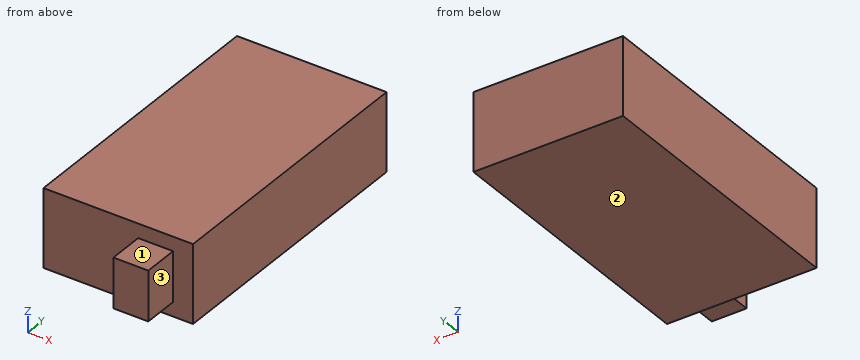
Autodesk Inventor part; units mm, degrees
ref_plane "Work Plane1" through (15.0814, 10.922, 0) normal (0, -1, 0) x (0, 0, -1)
ref_plane "XZ Plane" through (0, 0, 0) normal (0, 1, 0) x (-1, 0, 0)
sketch "Sketch1" plane through (0, 0, 0) normal (0, 0, 1) x (1, 0, 0)
  circle A0 centre (0, 0) radius 3.175
  line L0 (5.0349, -7.366) -> (-5.0349, -7.366)
  line L1 (-8.89, 10.922) -> (-8.89, -7.366)
  line L2 (8.89, -7.366) -> (8.89, 10.922)
  line L3 (-37.211, 10.922) -> (12.7, 10.922) construction
  line L4 (-8.89, 10.922) -> (8.89, 10.922)
  line L5 (8.89, 10.922) -> (8.89, -7.366)
  line L6 (8.89, -7.366) -> (-8.89, -7.366)
  line L7 (-8.89, -7.366) -> (-8.89, 10.922)
extrude "Extrusion1" add sketch "Sketch1" along normal mid plane 25.4 contours A0 | L0 L6 L1 L4 L2
ref_plane "Work Plane1" through (15.0814, 10.922, 0) normal (0, -1, 0) x (0, 0, -1)
sketch "Sketch3" plane through (15.0814, 10.922, 0) normal (0, -1, 0) x (0, 0, -1)
  line L0 (-19.939, 3.9686) -> (19.939, 3.9686)
  line L1 (19.939, 3.9686) -> (19.939, -72.2314)
  line L2 (19.939, -72.2314) -> (-19.939, -72.2314)
  line L3 (-19.939, -72.2314) -> (-19.939, 3.9686)
  line L4 (-9.525, 3.9686) -> (9.525, 3.9686) construction
  arc A0 (-19.939, -52.2924) -> (19.939, -52.2924) centre (0, -52.2924) ccw construction
  point P0 (0, -15.0814)
  point P1 (-19.939, -2.3814)
  point P2 (19.939, -2.3814)
extrude "Extrusion2" add sketch "Sketch3" against normal blind 142.705
properties part number "UpperArmActuatorBaseBoundingBox"
CAD build for the part. Positions are in the model's coordinates, mm. Face numbers are marked on the shaded views. A direction names the side the tool comes from. Round coordinates to 2 decimals unless told otherwise and drop trailing zeros. Loops run counter-clockwise (first coordinate to the right, second up) from the corner with the lowest first, then second, coordinate; pieces in that order, holes last. Notation, with made-up numbers: M 10,61 L 26,61 A11 cw 26,82 Z; hole C -19.5,49 d4. An arc over 180 degrees is marked long. One line per question, with ' | ' between items. Start each with the question number.
Item 1: Pin check, flat tips, straight feed: pin 1 Ø9 at (x, y) = (4, 4) entering from +Z; pin 2 Ø5.5 at (x, y) = (-0.5, 1) entering from -Z; pin 3 Ø9 at (y, z) = (2.5, 3) entering from -X. Stop position of each tip, or through.
Item 2: Cut at A-A, the plane x = -6. Write the cut outline in (y, z), plus the area to 3 significant figures.
Item 3: Cut at B-B, the plane z = 8. Write the cut outline in (x, y), plus the area to 3 significant figures.
Item 4: Wall check: line 1 (Y direction, x = -9, z = -1). Give the ranges that are in metal, low to high.
Item 5: Cut at C-C, the plane x = 14. Write the cut outline in (y, z).
Item 6: Which spindle directions (+Z, -Z, +X, -X, +Y, -Y) get a long thin tool onto all of the face, cutting with end or side? Do the marked faces 1, 2 and 3. Say none if no direction does.
Responses:
1) pin 1: stops at z = 12.7 | pin 2: stops at z = -12.7 | pin 3: stops at x = -8.89
2) outline: M -7.37,-12.7 L 10.92,-12.7 L 10.92,-19.94 L 153.63,-19.94 L 153.63,19.94 L 10.92,19.94 L 10.92,12.7 L -7.37,12.7 Z | area: 6,160 mm²
3) outline: M -57.15,10.92 L -8.89,10.92 L -8.89,-7.37 L 8.89,-7.37 L 8.89,10.92 L 19.05,10.92 L 19.05,153.63 L -57.15,153.63 Z | area: 11,200 mm²
4) line 1: y = 10.92 to 153.63
5) outline: M 10.92,-19.94 L 153.63,-19.94 L 153.63,19.94 L 10.92,19.94 Z
6) face 1: +Z, +X, -X, -Y | face 2: -Z, +X, -X, +Y, -Y | face 3: +Z, -Z, +X, -Y
